from build123d import *

# Parameters (mm, degrees)
F0_R     = 6.2452743357
F3_DEPTH = 10
F1_DEPTH = 15
F2_DEPTH = 6
F2_TAPER = -3
F4_R     = 0.351908714
F5_DEPTH = 7.938971743


with BuildPart() as f3:
    # F0 (on Front) → F3 (new body)
    with BuildSketch(Plane.XZ):
        with BuildLine():
            Line((11.1467493973, -12.6034934074), (1.9026910835, 17.1933302465))
            ThreePointArc((1.9026910835, 17.1933302465), (-0.0052668021, 18.6007195565), (-1.9163570551, 17.1975866305))
            Line((-1.9163570551, 17.1975866305), (-11.2346072181, -12.6034934074))
            Line((-11.2346072181, -12.6034934074), (11.1467493973, -12.6034934074))
        make_face()
        Circle(F0_R, mode=Mode.SUBTRACT)
        Circle(F0_R)
    extrude(amount=F3_DEPTH)

    # F0 (on Front) → F1 (join)
    with BuildSketch(Plane.XZ):
        Circle(F0_R)
    extrude(amount=F1_DEPTH)

    # F0 (on Front) → F2 (join)
    with BuildSketch(Plane.XZ):
        Circle(F0_R)
    extrude(amount=-F2_DEPTH, taper=F2_TAPER)

    # F4 (on face) → F5 (join)
    with BuildSketch(Plane.XZ):
        Circle(F4_R)
    extrude(amount=-F5_DEPTH)


solid = f3.part
Here's how the part is built. I have some questions about the finished solid (model axes, mm). A direction names the side the tool comes from. Coordinates: 2 decimals unless noted, no trailing zeros. Order: outer loops, then holes, each group sorted by start corner. A loop starts at its lowest first (then second) coordinate and runs counter-clockwise, first axis right, second up. Notation, with made-up numbers: (32, 30.25) - (89, 30.25) arc R28 ccw to (89, 49.25) - close; hole circle Ø11 at (49.5, 76). An arc over 180 degrees is marked (long way). Use CSV: the item, a comma, the result in double quotes. Start each with the question number.
1. Suppose I cut it at A-A on y = -0.75. List the corners of the cut face in (x, z) for me, then the cut area to 3 significant figures.
2. For faces 1 (the face through (6.076, 2.375, 1.913)), 2 (the face through (3.357, -12.465, 5.266)), 3 (the face through (-6.51, -4.93, 2.51)), which set-ups out of +Z, -Z, +X, -X, +Y, -Y let a thin tool reach every point of the face, with its end or its side?
3. Suppose I cut it at B-B on x = -7.5. List the corners of the cut face in (y, z) for me.
4. I'm going to push flat-ended pins straight in: pin 1 (8 mm diameter, centred on x = -2.5, y = 5, fed in from -Z); pin 2 (12 mm diameter, centred on y = -0.5, z = 0.5, fed in from +X); pin 3 (6.5 mm diameter, centred on x = 3, z = 2.5, fed in from +Y). Where does each tip first touch, or does it pass through?
5. Suppose I cut it at C-C on y = 5.5. List the corners of the cut face in (x, z) for me.
6. Please list where these lines run through material, in increasing order: line 1 (Y direction, x = -5.75, z = -7.5); line 2 (Y direction, x = -5.25, z = 0.5); line 3 (X direction, y = -5, z = -7.5). Write a range as from..to.
Output:
1,outline,"(-11.23, -12.6) - (11.15, -12.6) - (1.9, 17.19) arc R2 ccw to (-1.92, 17.2) - close"
1,area,"394 mm2"
2,face 1,"none"
2,face 2,"-Y"
2,face 3,"+Z, -X, +Y, -Y"
3,outline,"(-10, -12.6) - (0, -12.6) - (0, -0.66) - (-10, -0.66) - close"
4,pin 1,"stops at z = -6.56"
4,pin 2,"stops at x = 8.94"
4,pin 3,"stops at y = 6"
5,outline,"circle Ø13.07 at (0, 0)"
6,line 1,"y = -10..0"
6,line 2,"y = -15..6"
6,line 3,"x = -9.64..9.56"
